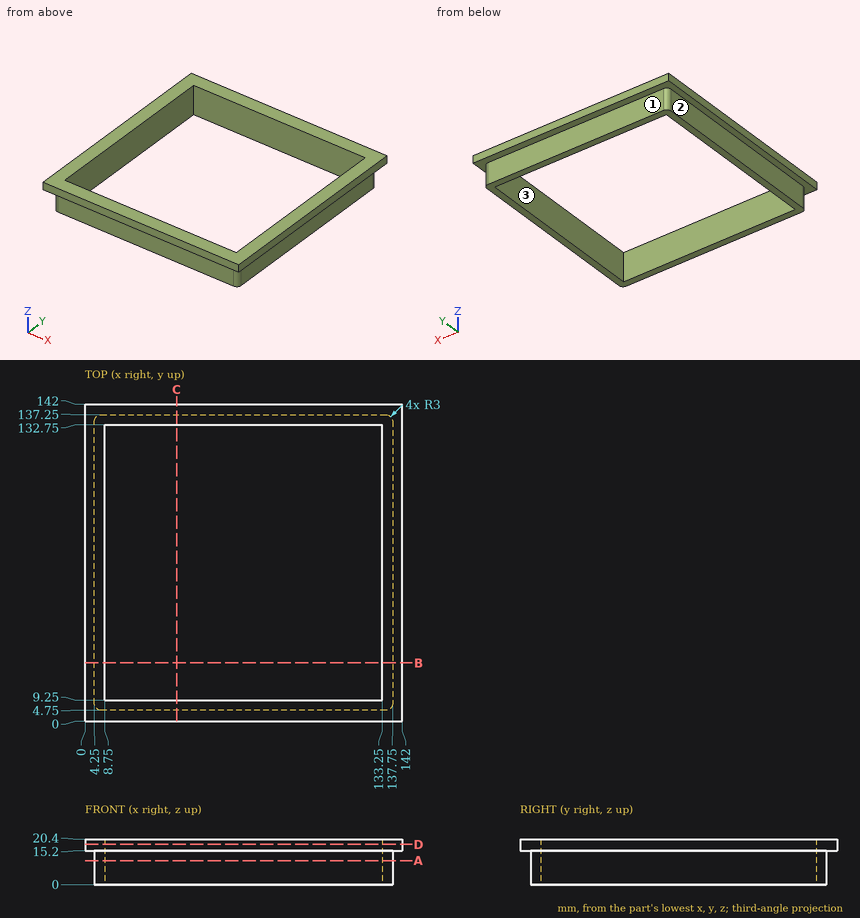
Part print with two shaded views. Sizes in mm from the minimum x, y, z corner. Give positions to 0.01 mm unless a question says otherwise; leave off trailing zeros. Order: outer loops, then holes, each group sorted by start corner. A loop starts at its lowest first (then second) coordinate and runs counter-clockwise, first axis right, second up.
1) Saw through at C-C, the plane x = 41. Write the cut outline in (y, z).
2) Wall check: probe 1 along X at (y, z) = (52, 19.25); probe 2 along Y at (x, z) = (117.5, 6); probe 3 along X at (y, z) = (49.5, 7.75). Give the ranges that are in metal, low to high.
3) Mould opens along Y. For the marked faces 1, 2 and 3 say: +Y half, -Y half, draft (parallel to the pull), parting line (faces both ways), or undercut.
4) Saw through at B-B, the plane y = 26. Write the cut outline in (x, z).
5) Pin check, flat tips, straight feed: pin 1 (1 mm diameter, centred on y = 51, z = 5, fed in from +X); pin 2 (4.5 mm diameter, centred on y = 93.5, z = 5, fed in from -X); pin 3 (5 mm diameter, centred on x = 15.5, z = 13, fed in from -Y); pin 4 (1 mm diameter, centred on x = 108.5, z = 5, fed in from +Y). Stop position of each tip, or through.
6) Saw through at D-D, the plane z = 18. Write the cut outline in (x, y).
7) Saw through at A-A, the plane z = 10.75. Write the cut outline in (x, y).
Computed:
1. outline: (0, 15.2) - (4.75, 15.2) - (4.75, 0) - (9.25, 0) - (9.25, 20.4) - (0, 20.4) - close; (132.75, 0) - (137.25, 0) - (137.25, 15.2) - (142, 15.2) - (142, 20.4) - (132.75, 20.4) - close
2. probe 1: x = 0 to 8.75, 133.25 to 142
2. probe 2: y = 4.75 to 9.25, 132.75 to 137.25
2. probe 3: x = 4.25 to 8.75, 133.25 to 137.75
3. face 1: +Y half
3. face 2: draft
3. face 3: undercut
4. outline: (0, 15.2) - (4.25, 15.2) - (4.25, 0) - (8.75, 0) - (8.75, 20.4) - (0, 20.4) - close; (133.25, 0) - (137.75, 0) - (137.75, 15.2) - (142, 15.2) - (142, 20.4) - (133.25, 20.4) - close
5. pin 1: stops at x = 137.75
5. pin 2: stops at x = 4.25
5. pin 3: stops at y = 0
5. pin 4: stops at y = 137.25
6. outline: (0, 0) - (142, 0) - (142, 142) - (0, 142) - close; hole (8.75, 9.25) - (133.25, 9.25) - (133.25, 132.75) - (8.75, 132.75) - close
7. outline: (4.25, 7.75) arc R3 ccw to (7.25, 4.75) - (134.75, 4.75) arc R3 ccw to (137.75, 7.75) - (137.75, 134.25) arc R3 ccw to (134.75, 137.25) - (7.25, 137.25) arc R3 ccw to (4.25, 134.25) - close; hole (8.75, 9.25) - (133.25, 9.25) - (133.25, 132.75) - (8.75, 132.75) - close
